Geometry check sheet. Reference: the model listing, model coordinates, mm. Face numbers are marked on the shaded views. Round coordinates to 2 decimals unless told otherwise and drop trailing zeros. Order: outer loops, then holes, each group sorted by start corner. A loop starts at its lowest first (then second) coordinate and runs counter-clockwise, first axis right, second up.
(1) Material ranges on line 1 along Z through (x, y) = (88.5, -37); line 2 along Y through (x, z) = (-86, 154); line 3 along Y through (x, z) = (0, 208), recorded low to high.
(2) Sectioned sample at C-C (y = -17.5). Give the number of separate pieces and of enclosed holes in the cut face, plus the area to 3 significant figures.
(3) Sectioned sample at A-A (z = 125.5). Record the boundary of the cut face in (x, y).
(4) Go/stop test with flat-tipped pins: pin 1 (5 mm diameter, centred on y = 86.5, z = 65.5, fed in from -X); pin 2 (19 mm diameter, centred on x = -13, y = -87.5, fed in from +Z); pin 3 (8.5 mm diameter, centred on y = 85, z = 101.5, fed in from +X). Record where each tip stops, or that it passes through.
(5) Sectioned sample at B-B (x = 66.5). Record the boundary of the cut face in (y, z), plus the area to 3 significant figures.
(6) Release check for a two-part mould opening along X. For the marked faces 1 and 2 record: +X half, -X half, draft (parallel to the pull), parting line (faces both ways), or undercut.
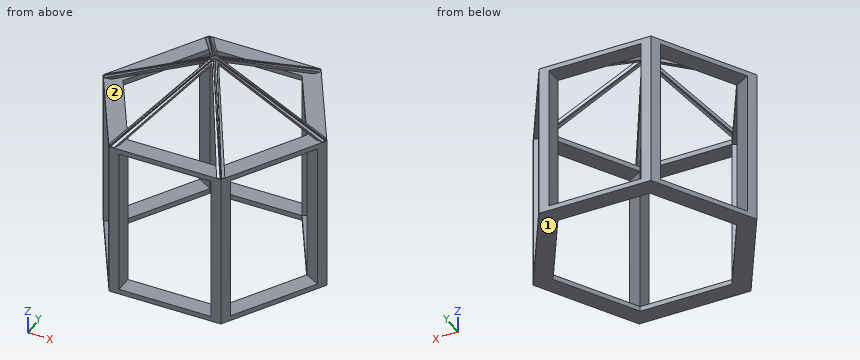
from build123d import *

# Parameters (mm, degrees)
CYLINDER_R                  = 4.5
CYLINDER_DEPTH              = 1000
PAD004_DEPTH                = 3
BODY004_PLACEMENT_ANGLE     = 60
PAD003_DEPTH                = 3
BODY003_PLACEMENT_ANGLE     = 60
PAD006_DEPTH                = 3
BODY006_PLACEMENT_ANGLE     = 60
PAD005_DEPTH                = 3
BODY005_PLACEMENT_ANGLE     = 60
CUT003_PLACEMENT_ANGLE      = 60
PAD008_DEPTH                = 3
BODY008_PLACEMENT_ANGLE     = 60
PAD007_DEPTH                = 3
BODY007_PLACEMENT_ANGLE     = 60
CUT004_PLACEMENT_ANGLE      = 120
PAD010_DEPTH                = 3
BODY010_PLACEMENT_ANGLE     = 60
PAD009_DEPTH                = 3
BODY009_PLACEMENT_ANGLE     = 60
CUT005_PLACEMENT_ANGLE      = 180
PAD012_DEPTH                = 3
BODY012_PLACEMENT_ANGLE     = 60
PAD011_DEPTH                = 3
BODY011_PLACEMENT_ANGLE     = 60
CUT006_PLACEMENT_ANGLE      = 240
PAD014_DEPTH                = 3
BODY014_PLACEMENT_ANGLE     = 60
PAD013_DEPTH                = 3
BODY013_PLACEMENT_ANGLE     = 60
CUT007_PLACEMENT_ANGLE      = 300
BOX_W                       = 92.4
BOX_H                       = 18
BOX_DEPTH                   = 147
BOX001_W                    = 92.4
BOX001_H                    = 18
BOX001_DEPTH                = 147
COMPOUND001_PLACEMENT_ANGLE = 60
BOX002_W                    = 92.4
BOX002_H                    = 18
BOX002_DEPTH                = 147
COMPOUND002_PLACEMENT_ANGLE = 120
BOX003_W                    = 92.4
BOX003_H                    = 18
BOX003_DEPTH                = 147
COMPOUND003_PLACEMENT_ANGLE = 180
BOX004_W                    = 92.4
BOX004_H                    = 18
BOX004_DEPTH                = 147
COMPOUND004_PLACEMENT_ANGLE = 240
BOX005_W                    = 92.4
BOX005_H                    = 18
BOX005_DEPTH                = 147
COMPOUND005_PLACEMENT_ANGLE = 300
PAD001_DEPTH                = 157
PAD_DEPTH                   = 157


with BuildPart() as cylinder:
    # Cylinder → Cylinder (new body)
    with BuildSketch(Plane.XY):
        Circle(CYLINDER_R)
    extrude(amount=CYLINDER_DEPTH)


with BuildPart() as compound007:
    # Sketch004 → Pad004 (new body)
    with BuildSketch(Plane.XZ):
        Polygon((-51.5, 0), (51.5, 0), (0, 105), align=None)
    extrude(amount=PAD004_DEPTH)


with BuildPart() as compound007_1:
    # Body004 placement: moved
    add(compound007.part.moved(Location((0, 96.6, 157))).rotate(Axis((0, 96.6, 157), (1, 0, 0)), BODY004_PLACEMENT_ANGLE))


with BuildPart() as cut002:
    # Sketch003 → Pad003 (new body)
    with BuildSketch(Plane.XZ):
        Polygon((-56.5, 0), (56.5, 0), (0, 115), align=None)
    extrude(amount=PAD003_DEPTH)


with BuildPart() as cut002_1:
    # Body003 placement: moved
    add(cut002.part.moved(Location((0, 96.6, 157))).rotate(Axis((0, 96.6, 157), (1, 0, 0)), BODY003_PLACEMENT_ANGLE))

    # Cut002: cut Compound007
    add(compound007_1.part, mode=Mode.SUBTRACT)


with BuildPart() as compound009:
    # Sketch006 → Pad006 (new body)
    with BuildSketch(Plane.XZ):
        Polygon((-51.5, 0), (51.5, 0), (0, 105), align=None)
    extrude(amount=PAD006_DEPTH)


with BuildPart() as compound009_1:
    # Body006 placement: moved
    add(compound009.part.moved(Location((0, 96.6, 157))).rotate(Axis((0, 96.6, 157), (1, 0, 0)), BODY006_PLACEMENT_ANGLE))


with BuildPart() as cut003:
    # Sketch005 → Pad005 (new body)
    with BuildSketch(Plane.XZ):
        Polygon((-56.5, 0), (56.5, 0), (0, 115), align=None)
    extrude(amount=PAD005_DEPTH)


with BuildPart() as cut003_1:
    # Body005 placement: moved
    add(cut003.part.moved(Location((0, 96.6, 157))).rotate(Axis((0, 96.6, 157), (1, 0, 0)), BODY005_PLACEMENT_ANGLE))

    # Cut003: cut Compound009
    add(compound009_1.part, mode=Mode.SUBTRACT)


with BuildPart() as cut003_2:
    # Cut003 placement: moved
    add(cut003_1.part.rotate(Axis((0, 0, 0), (0, 0, 1)), CUT003_PLACEMENT_ANGLE))


with BuildPart() as compound011:
    # Sketch008 → Pad008 (new body)
    with BuildSketch(Plane.XZ):
        Polygon((-51.5, 0), (51.5, 0), (0, 105), align=None)
    extrude(amount=PAD008_DEPTH)


with BuildPart() as compound011_1:
    # Body008 placement: moved
    add(compound011.part.moved(Location((0, 96.6, 157))).rotate(Axis((0, 96.6, 157), (1, 0, 0)), BODY008_PLACEMENT_ANGLE))


with BuildPart() as cut004:
    # Sketch007 → Pad007 (new body)
    with BuildSketch(Plane.XZ):
        Polygon((-56.5, 0), (56.5, 0), (0, 115), align=None)
    extrude(amount=PAD007_DEPTH)


with BuildPart() as cut004_1:
    # Body007 placement: moved
    add(cut004.part.moved(Location((0, 96.6, 157))).rotate(Axis((0, 96.6, 157), (1, 0, 0)), BODY007_PLACEMENT_ANGLE))

    # Cut004: cut Compound011
    add(compound011_1.part, mode=Mode.SUBTRACT)


with BuildPart() as cut004_2:
    # Cut004 placement: moved
    add(cut004_1.part.rotate(Axis((0, 0, 0), (0, 0, 1)), CUT004_PLACEMENT_ANGLE))


with BuildPart() as compound013:
    # Sketch010 → Pad010 (new body)
    with BuildSketch(Plane.XZ):
        Polygon((-51.5, 0), (51.5, 0), (0, 105), align=None)
    extrude(amount=PAD010_DEPTH)


with BuildPart() as compound013_1:
    # Body010 placement: moved
    add(compound013.part.moved(Location((0, 96.6, 157))).rotate(Axis((0, 96.6, 157), (1, 0, 0)), BODY010_PLACEMENT_ANGLE))


with BuildPart() as cut005:
    # Sketch009 → Pad009 (new body)
    with BuildSketch(Plane.XZ):
        Polygon((-56.5, 0), (56.5, 0), (0, 115), align=None)
    extrude(amount=PAD009_DEPTH)


with BuildPart() as cut005_1:
    # Body009 placement: moved
    add(cut005.part.moved(Location((0, 96.6, 157))).rotate(Axis((0, 96.6, 157), (1, 0, 0)), BODY009_PLACEMENT_ANGLE))

    # Cut005: cut Compound013
    add(compound013_1.part, mode=Mode.SUBTRACT)


with BuildPart() as cut005_2:
    # Cut005 placement: moved
    add(cut005_1.part.rotate(Axis((0, 0, 0), (0, 0, 1)), CUT005_PLACEMENT_ANGLE))


with BuildPart() as compound015:
    # Sketch012 → Pad012 (new body)
    with BuildSketch(Plane.XZ):
        Polygon((-51.5, 0), (51.5, 0), (0, 105), align=None)
    extrude(amount=PAD012_DEPTH)


with BuildPart() as compound015_1:
    # Body012 placement: moved
    add(compound015.part.moved(Location((0, 96.6, 157))).rotate(Axis((0, 96.6, 157), (1, 0, 0)), BODY012_PLACEMENT_ANGLE))


with BuildPart() as cut006:
    # Sketch011 → Pad011 (new body)
    with BuildSketch(Plane.XZ):
        Polygon((-56.5, 0), (56.5, 0), (0, 115), align=None)
    extrude(amount=PAD011_DEPTH)


with BuildPart() as cut006_1:
    # Body011 placement: moved
    add(cut006.part.moved(Location((0, 96.6, 157))).rotate(Axis((0, 96.6, 157), (1, 0, 0)), BODY011_PLACEMENT_ANGLE))

    # Cut006: cut Compound015
    add(compound015_1.part, mode=Mode.SUBTRACT)


with BuildPart() as cut006_2:
    # Cut006 placement: moved
    add(cut006_1.part.rotate(Axis((0, 0, 0), (0, 0, 1)), CUT006_PLACEMENT_ANGLE))


with BuildPart() as compound017:
    # Sketch014 → Pad014 (new body)
    with BuildSketch(Plane.XZ):
        Polygon((-51.5, 0), (51.5, 0), (0, 105), align=None)
    extrude(amount=PAD014_DEPTH)


with BuildPart() as compound017_1:
    # Body014 placement: moved
    add(compound017.part.moved(Location((0, 96.6, 157))).rotate(Axis((0, 96.6, 157), (1, 0, 0)), BODY014_PLACEMENT_ANGLE))


with BuildPart() as cut008:
    # Sketch013 → Pad013 (new body)
    with BuildSketch(Plane.XZ):
        Polygon((-56.5, 0), (56.5, 0), (0, 115), align=None)
    extrude(amount=PAD013_DEPTH)


with BuildPart() as cut008_1:
    # Body013 placement: moved
    add(cut008.part.moved(Location((0, 96.6, 157))).rotate(Axis((0, 96.6, 157), (1, 0, 0)), BODY013_PLACEMENT_ANGLE))

    # Cut007: cut Compound017
    add(compound017_1.part, mode=Mode.SUBTRACT)


with BuildPart() as cut008_2:
    # Cut007 placement: moved
    add(cut008_1.part.rotate(Axis((0, 0, 0), (0, 0, 1)), CUT007_PLACEMENT_ANGLE))

    # Fusion001: union Cut002, Cut003, Cut004, Cut005, Cut006
    add(cut002_1.part)
    add(cut003_2.part)
    add(cut004_2.part)
    add(cut005_2.part)
    add(cut006_2.part)

    # Cut008: cut Cylinder
    add(cylinder.part, mode=Mode.SUBTRACT)


with BuildPart() as compound:
    # Box → Box (new body)
    with BuildSketch(Plane(origin=(-46.2, 80, 5), x_dir=(1, 0, 0), z_dir=(0, 0, 1))):
        with Locations((46.2, 9)):
            Rectangle(BOX_W, BOX_H)
    extrude(amount=BOX_DEPTH)


with BuildPart() as compound001:
    # Box001 → Box001 (new body)
    with BuildSketch(Plane(origin=(-46.2, 80, 5), x_dir=(1, 0, 0), z_dir=(0, 0, 1))):
        with Locations((46.2, 9)):
            Rectangle(BOX001_W, BOX001_H)
    extrude(amount=BOX001_DEPTH)


with BuildPart() as compound001_1:
    # Compound001 placement: moved
    add(compound001.part.rotate(Axis((0, 0, 0), (0, 0, 1)), COMPOUND001_PLACEMENT_ANGLE))


with BuildPart() as compound002:
    # Box002 → Box002 (new body)
    with BuildSketch(Plane(origin=(-46.2, 80, 5), x_dir=(1, 0, 0), z_dir=(0, 0, 1))):
        with Locations((46.2, 9)):
            Rectangle(BOX002_W, BOX002_H)
    extrude(amount=BOX002_DEPTH)


with BuildPart() as compound002_1:
    # Compound002 placement: moved
    add(compound002.part.rotate(Axis((0, 0, 0), (0, 0, 1)), COMPOUND002_PLACEMENT_ANGLE))


with BuildPart() as compound003:
    # Box003 → Box003 (new body)
    with BuildSketch(Plane(origin=(-46.2, 80, 5), x_dir=(1, 0, 0), z_dir=(0, 0, 1))):
        with Locations((46.2, 9)):
            Rectangle(BOX003_W, BOX003_H)
    extrude(amount=BOX003_DEPTH)


with BuildPart() as compound003_1:
    # Compound003 placement: moved
    add(compound003.part.rotate(Axis((0, 0, 0), (0, 0, 1)), COMPOUND003_PLACEMENT_ANGLE))


with BuildPart() as compound004:
    # Box004 → Box004 (new body)
    with BuildSketch(Plane(origin=(-46.2, 80, 5), x_dir=(1, 0, 0), z_dir=(0, 0, 1))):
        with Locations((46.2, 9)):
            Rectangle(BOX004_W, BOX004_H)
    extrude(amount=BOX004_DEPTH)


with BuildPart() as compound004_1:
    # Compound004 placement: moved
    add(compound004.part.rotate(Axis((0, 0, 0), (0, 0, 1)), COMPOUND004_PLACEMENT_ANGLE))


with BuildPart() as fusion:
    # Box005 → Box005 (new body)
    with BuildSketch(Plane(origin=(-46.2, 80, 5), x_dir=(1, 0, 0), z_dir=(0, 0, 1))):
        with Locations((46.2, 9)):
            Rectangle(BOX005_W, BOX005_H)
    extrude(amount=BOX005_DEPTH)


with BuildPart() as fusion_1:
    # Compound005 placement: moved
    add(fusion.part.rotate(Axis((0, 0, 0), (0, 0, 1)), COMPOUND005_PLACEMENT_ANGLE))

    # Fusion: union Compound, Compound001, Compound002, Compound003, Compound004
    add(compound.part)
    add(compound001_1.part)
    add(compound002_1.part)
    add(compound003_1.part)
    add(compound004_1.part)


with BuildPart() as body001:
    # Sketch001 → Pad001 (new body)
    with BuildSketch(Plane.XY):
        Polygon((92.4, 0), (46.2, 80.020747), (-46.2, 80.020747), (-92.4, 0), (-46.2, -80.020747), (46.2, -80.020747), align=None)
    extrude(amount=PAD001_DEPTH)


with BuildPart() as fusion002:
    # Sketch → Pad (new body)
    with BuildSketch(Plane.XY):
        Polygon((112.4, 0), (56.2, 97.341255), (-56.2, 97.341255), (-112.4, 0), (-56.2, -97.341255), (56.2, -97.341255), align=None)
    extrude(amount=PAD_DEPTH)

    # Cut: cut Body001
    add(body001.part, mode=Mode.SUBTRACT)

    # Cut001: cut Fusion
    add(fusion_1.part, mode=Mode.SUBTRACT)

    # Fusion002: union Cut008
    add(cut008_2.part)


solid = fusion002.part
Answer below:
1. line 1: z = 0 to 5, 152 to 157
1. line 2: y = -45.73 to -11.09, 11.09 to 45.73
1. line 3: y = -4.8 to -4.5, 4.5 to 4.8
2. separate pieces: 6
2. enclosed holes: 0
2. area: 444 mm2
3. outline: (-112.4, 0) - (-107.4, -8.66) - (-92.4, 0) - (-107.4, 8.66) - close; (-61.2, -88.68) - (-56.2, -97.34) - (-46.2, -97.34) - (-46.2, -80.02) - close; (-61.2, 88.68) - (-46.2, 80.02) - (-46.2, 97.34) - (-56.2, 97.34) - close; (46.2, -97.34) - (56.2, -97.34) - (61.2, -88.68) - (46.2, -80.02) - close; (46.2, 80.02) - (61.2, 88.68) - (56.2, 97.34) - (46.2, 97.34) - close; (92.4, 0) - (107.4, -8.66) - (112.4, 0) - (107.4, 8.66) - close
4. pin 1: stops at x = -61.2
4. pin 2: stops at z = 157
4. pin 3: stops at x = 61.2
5. outline: (-79.5, 0) - (-44.86, 0) - (-44.86, 5) - (-79.5, 5) - close; (-79.5, 152) - (-44.86, 152) - (-44.86, 157) - (-79.5, 157) - close; (-3.34, 178.56) - (-2.6, 175.31) - (0, 176.06) - (2.6, 175.31) - (3.34, 178.56) - (1.11, 179.2) - (0.97, 179.8) - (0, 179.52) - (-0.97, 179.8) - (-1.11, 179.2) - close; (44.86, 0) - (79.5, 0) - (79.5, 5) - (44.86, 5) - close; (44.86, 152) - (79.5, 152) - (79.5, 157) - (44.86, 157) - close
5. area: 714 mm2
6. face 1: draft
6. face 2: undercut
